Source: three-view drawing plus pictorial views. Frame: mm from the lowest corner of the part. Give positions to 0.01 mm unless a question says otherwise; leave off trailing zeros. Loops run counter-clockwise (first coordinate to the right, second up) from the corner with the lowest first, then second, coordinate; pieces in that order, holes last. Notation, with made-up numbers: (-16.5, 13.5) -> (38.5, 13.5) arc R30 cw to (38.5, 44.5) -> close; hole circle Ø9 at (1, 60.5). An arc over 180 degrees is marked (long way). Answer as a JSON object with one key per item and string values. Group by question number.
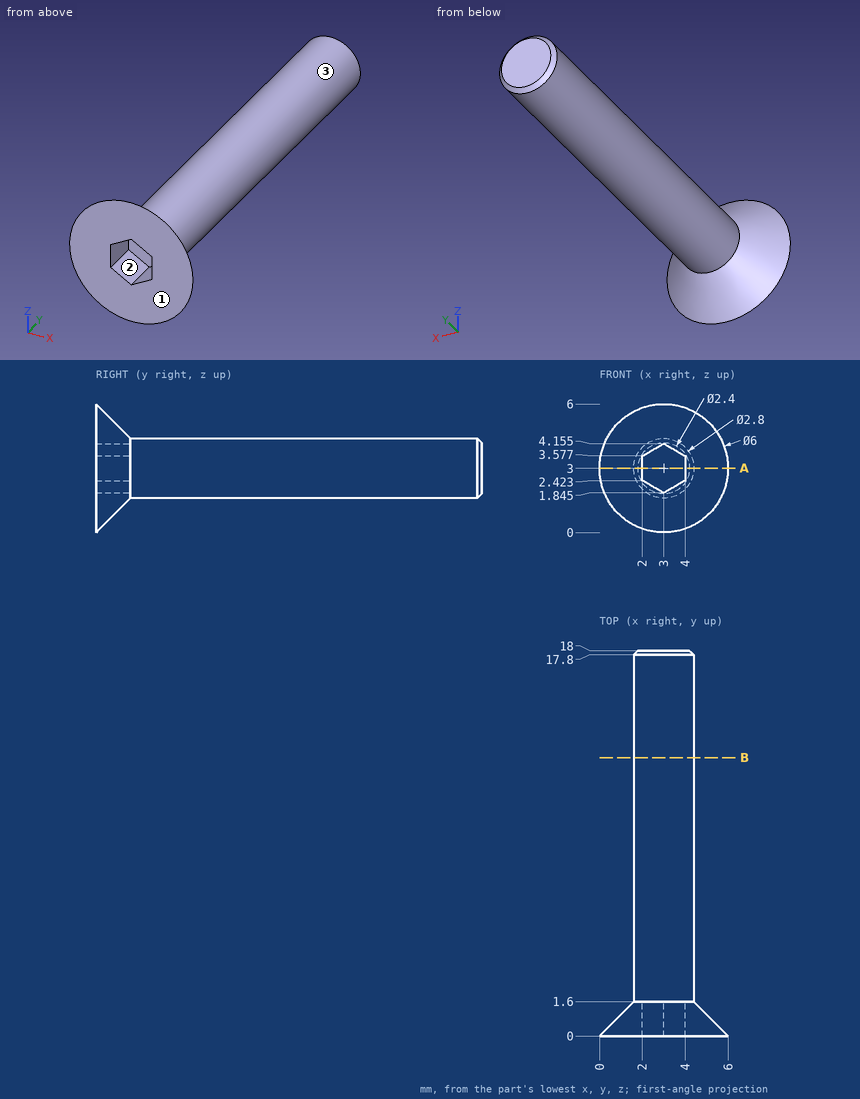
(1) First-contact query: pin 1 (2 mm diameter, centred on x = 1, z = 4, fed in from +Y) (1 decimal); pin 2 (1 mm diameter, centred on x = 5, z = 4.5, fed in from +Y); pin 3 (0.9 mm diameter, centred on y = 1, z = 3, fed in from -X). Flat tips, straight axial feed; report the tip coordinate or a pass-through.
(2) Material intervals for line 1 (Z direction, x = 2.5, y = 1.25) (1 decimal); line 2 (Z direction, x = 3.4, y = 1.5) (1 decimal); line 3 (X direction, y = 1, z = 3.25) (1 decimal), sorted ascending. Write a range as from..to.
(3) Section query A-A on z = 3. Return the cut outline in (x, y).
(4) Section query B-B on y = 13. Return the cut outline in (x, z).
(5) Mould query, pull axis Z, two halves, no side actions, for the marked faces 1, 2 and 3. Classes: pulls with the +Z half, pulls with the -Z half, needs draft (parallel to the pull), parting line crosses it, or undercut.
Result:
{
 "1": {"pin 1": "y = 18", "pin 2": "y = 1", "pin 3": "x = 0.55"},
 "2": {"line 1": "1.3..2.1, 3.9..4.7", "line 2": "1.6..2.1, 3.9..4.4", "line 3": "1..2, 4..5"},
 "3": {"outline": "(0, 0) -> (2, 0) -> (2, 1.6) -> (4, 1.6) -> (4, 0) -> (6, 0) -> (4.4, 1.6) -> (4.4, 17.8) -> (4.2, 18) -> (1.8, 18) -> (1.6, 17.8) -> (1.6, 1.6) -> close"},
 "4": {"outline": "circle Ø2.8 at (3, 3)"},
 "5": {"face 1": "needs draft", "face 2": "undercut", "face 3": "parting line crosses it"}
}
